For this review, take the finished solid that the model builds, in its own axes (mm). Face numbers are marked on the shaded views. A direction names the side the tool comes from. Give positions to 0.01 mm unless a question says otherwise; leave off trailing zeros. Loops run counter-clockwise (first coordinate to the right, second up) from the corner with the lowest first, then second, coordinate; pieces in that order, holes last. Notation, with made-up numbers: (-9, 53.5) -> (4, 53.5) arc R10 ccw to (4, 64.5) -> close; hole circle Ø7 at (-5.75, 61). An arc over 180 degrees is marked (long way). Answer as CSV lines item,"result". Start each with the question number.
Item 1: Add section C-C on y = -9.5. State the section outline as (x, z) points.
Item 2: For L1, parallel to X at y = 8.5, z = 25; L2, parallel to X at y = -9.5, z = 46; L3, parallel to Y at x = -40, z = 10, list the stretches that pass through material, from the lowest coordinate up. Write a range as from..to.
Item 3: Machinability: for the marked faces 1, 2 and 3, which of the approach directions +Z, -Z, +X, -X, +Y, -Y give a long, thin tool a straight path to every point of the face, cutting with its end or side? Answer none if there is none.
Item 4: The part is to be moulded in two halves that separate along Z. For the marked faces 4, 5 and 6, say which applies: +Z half, -Z half, draft (parallel to the pull), parting line (faces both ways), or undercut.
Item 5: Clearance check with flat-ended pins moving along their axes: P1, Ø4.5, axis at y = 0, z = 10, coming from the -X side; P2, Ø8, axis at y = -15, z = 25, coming from the +X side. State where each tip first meets the part, or that it passes through.
Item 6: Add section A-A on z = 25. State the section outline as (x, y) points.
Item 7: Add section B-B on y = 0. State the section outline as (x, z) points.
Item 8: Add section D-D on x = -16. State the section outline as (y, z) points.
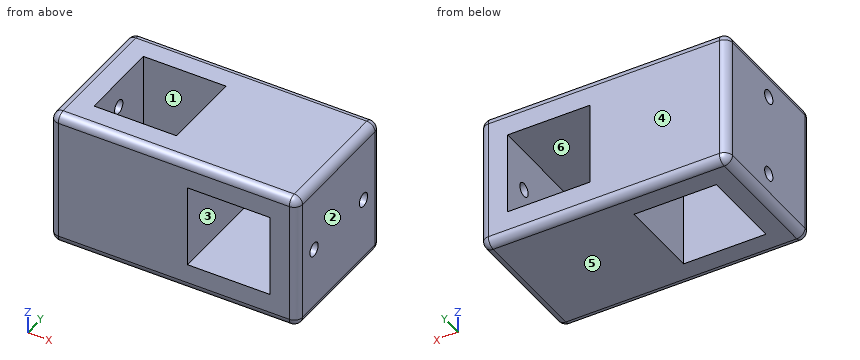
```python
from build123d import *

# Parameters (mm, degrees)
SKETCH1_W           = 90
SKETCH1_H           = 50
BOSS_EXTRUDE1_DEPTH = 50
CUT_EXTRUDE1_REACH  = 52
SKETCH2_W           = 30
SKETCH2_H           = 30
CUT_EXTRUDE2_REACH  = 52
SKETCH3_W           = 30
SKETCH3_H           = 30
FILLET1_R           = 3
CUT_EXTRUDE3_REACH  = 92
SKETCH4_R           = 2.5
CUT_EXTRUDE4_REACH  = 92
SKETCH5_R           = 2.5


with BuildPart() as part:
    # Sketch1 → Boss-Extrude1 (new body)
    with BuildSketch(Plane.XY):
        Rectangle(SKETCH1_W, SKETCH1_H)
    extrude(amount=BOSS_EXTRUDE1_DEPTH)

    # Sketch2 → Cut-Extrude1 (cut, up to next)
    with BuildSketch(Plane.XY.offset(50), mode=Mode.PRIVATE) as cut_extrude1_sk1:
        with Locations((-20, 0)):
            Rectangle(SKETCH2_W, SKETCH2_H)
    cut_extrude1_tool1 = extrude(cut_extrude1_sk1.sketch, amount=-CUT_EXTRUDE1_REACH, mode=Mode.PRIVATE) & part.part
    add(cut_extrude1_tool1.solids().sort_by_distance((-20, 0, 50))[0], mode=Mode.SUBTRACT)

    # Sketch3 → Cut-Extrude2 (cut, up to next)
    with BuildSketch(Plane(origin=(0, 25, 0), x_dir=(1, 0, 0), z_dir=(0, 1, 0)), mode=Mode.PRIVATE) as cut_extrude2_sk1:
        with Locations((20, -25)):
            Rectangle(SKETCH3_W, SKETCH3_H)
    cut_extrude2_tool1 = extrude(cut_extrude2_sk1.sketch, amount=-CUT_EXTRUDE2_REACH, mode=Mode.PRIVATE) & part.part
    add(cut_extrude2_tool1.solids().sort_by_distance((20, 25, 25))[0], mode=Mode.SUBTRACT)

    # Fillet1
    fillet1_edges = [part.edges().sort_by_distance(p)[0] for p in [
        (45, 0, 50),
        (0, 25, 50),
        (-45, 0, 50),
        (0, 25, 0),
        (45, 0, 0),
        (0, -25, 0),
        (-45, 0, 0),
        (-45, 25, 25),
        (45, 25, 25),
        (45, -25, 25),
        (-45, -25, 25),
        (0, -25, 50),
    ]]
    fillet(fillet1_edges, radius=FILLET1_R)

    # Sketch4 → Cut-Extrude3 (cut, up to next)
    with BuildSketch(Plane.ZY.offset(45), mode=Mode.PRIVATE) as cut_extrude3_sk1:
        with Locations((10, 0)):
            Circle(SKETCH4_R)
    cut_extrude3_tool1 = extrude(cut_extrude3_sk1.sketch, amount=-CUT_EXTRUDE3_REACH, mode=Mode.PRIVATE) & part.part
    add(cut_extrude3_tool1.solids().sort_by_distance((-45, 0, 10))[0], mode=Mode.SUBTRACT)
    # Sketch4 → Cut-Extrude3 (cut, up to next)
    with BuildSketch(Plane.ZY.offset(45), mode=Mode.PRIVATE) as cut_extrude3_sk2:
        with Locations((40, 0)):
            Circle(SKETCH4_R)
    cut_extrude3_tool2 = extrude(cut_extrude3_sk2.sketch, amount=-CUT_EXTRUDE3_REACH, mode=Mode.PRIVATE) & part.part
    add(cut_extrude3_tool2.solids().sort_by_distance((-45, 0, 40))[0], mode=Mode.SUBTRACT)

    # Sketch5 → Cut-Extrude4 (cut, up to next)
    with BuildSketch(Plane(origin=(45, 0, 0), x_dir=(0, 0, -1), z_dir=(1, 0, 0)), mode=Mode.PRIVATE) as cut_extrude4_sk1:
        with Locations((-25, 15)):
            Circle(SKETCH5_R)
    cut_extrude4_tool1 = extrude(cut_extrude4_sk1.sketch, amount=-CUT_EXTRUDE4_REACH, mode=Mode.PRIVATE) & part.part
    add(cut_extrude4_tool1.solids().sort_by_distance((45, 15, 25))[0], mode=Mode.SUBTRACT)
    # Sketch5 → Cut-Extrude4 (cut, up to next)
    with BuildSketch(Plane(origin=(45, 0, 0), x_dir=(0, 0, -1), z_dir=(1, 0, 0)), mode=Mode.PRIVATE) as cut_extrude4_sk2:
        with Locations((-25, -15)):
            Circle(SKETCH5_R)
    cut_extrude4_tool2 = extrude(cut_extrude4_sk2.sketch, amount=-CUT_EXTRUDE4_REACH, mode=Mode.PRIVATE) & part.part
    add(cut_extrude4_tool2.solids().sort_by_distance((45, -15, 25))[0], mode=Mode.SUBTRACT)


solid = part.part
```
Computed values:
1,outline,"(-45, 3) arc R3 ccw to (-42, 0) -> (-35, 0) -> (-35, 50) -> (-42, 50) arc R3 ccw to (-45, 47) -> close; (-5, 0) -> (42, 0) arc R3 ccw to (45, 3) -> (45, 47) arc R3 ccw to (42, 50) -> (-5, 50) -> close; hole (5, 10) -> (35, 10) -> (35, 40) -> (5, 40) -> close"
2,L1,"-45..-35, -5..5, 35..45"
2,L2,"-45..-35, -5..45"
2,L3,"-25..-2.5, 2.5..25"
3,face 1,"+Z, -Z"
3,face 2,"+Z, -Z, +X, +Y, -Y"
3,face 3,"+Y, -Y"
4,face 4,"draft"
4,face 5,"-Z half"
4,face 6,"undercut"
5,P1,"x = -5"
5,P2,"x = 45"
6,outline,"(-45, -22) arc R3 ccw to (-42, -25) -> (5, -25) -> (5, 25) -> (-42, 25) arc R3 ccw to (-45, 22) -> close; (35, -25) -> (42, -25) arc R3 ccw to (45, -22) -> (45, -17.5) -> (35, -17.5) -> close; (35, -12.5) -> (45, -12.5) -> (45, 12.5) -> (35, 12.5) -> close; (35, 17.5) -> (45, 17.5) -> (45, 22) arc R3 ccw to (42, 25) -> (35, 25) -> close; hole (-35, -15) -> (-5, -15) -> (-5, 15) -> (-35, 15) -> close"
7,outline,"(-45, 3) arc R3 ccw to (-42, 0) -> (-35, 0) -> (-35, 7.5) -> (-45, 7.5) -> close; (-45, 12.5) -> (-35, 12.5) -> (-35, 37.5) -> (-45, 37.5) -> close; (-45, 42.5) -> (-35, 42.5) -> (-35, 50) -> (-42, 50) arc R3 ccw to (-45, 47) -> close; (-5, 0) -> (42, 0) arc R3 ccw to (45, 3) -> (45, 47) arc R3 ccw to (42, 50) -> (-5, 50) -> close; hole (5, 10) -> (35, 10) -> (35, 40) -> (5, 40) -> close"
8,outline,"(-25, 3) arc R3 ccw to (-22, 0) -> (-15, 0) -> (-15, 50) -> (-22, 50) arc R3 ccw to (-25, 47) -> close; (15, 0) -> (22, 0) arc R3 ccw to (25, 3) -> (25, 47) arc R3 ccw to (22, 50) -> (15, 50) -> close"
